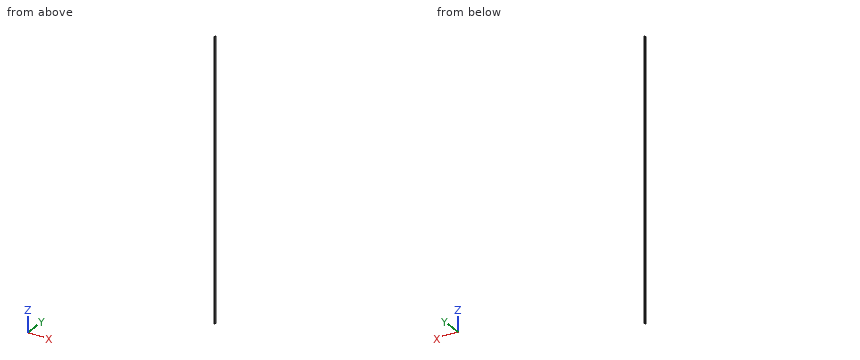
Autodesk Inventor part; units mm, degrees
ref_plane "Work Plane1" through (-1.2283, 0, 317.5) normal (0, 0, 1) x (1, 0, 0)
ref_plane "YZ Plane" through (0, 0, 0) normal (1, 0, 0) x (0, 1, 0)
ref_plane "XZ Plane" through (0, 0, 0) normal (0, 1, 0) x (-1, 0, 0)
ref_plane "Work Plane1" through (-1.2283, 0, 317.5) normal (0, 0, 1) x (1, 0, 0)
sketch "Sketch1" plane through (-1.2283, 0, 317.5) normal (0, 0, 1) x (1, 0, 0)
  line L0 (-0.3592, 8.7122) -> (-0.3592, 0.3592)
  line L1 (-0.3592, 0.3592) -> (0, 0)
  line L2 (0, 0) -> (2.4566, 0)
  line L3 (2.4566, 0) -> (2.8158, 0.3592)
  line L4 (2.8158, 0.3592) -> (2.8158, 7.6708)
  line L5 (2.8158, 7.6708) -> (2.6888, 7.6708)
  arc A0 (2.6888, 7.9248) -> (2.6888, 7.6708) centre (2.6888, 7.7978) ccw
  line L6 (2.6888, 7.9248) -> (4.3906, 7.9248)
  line L7 (4.3906, 7.9248) -> (4.3906, 8.7376)
  line L8 (4.3906, 8.7376) -> (2.2824, 10.8458)
  line L9 (2.2824, 10.8458) -> (1.7744, 10.8458)
  line L10 (1.7744, 10.8458) -> (-0.3592, 8.7122)
  point P0 (1.2283, 0)
extrude "Extrusion1" add sketch "Sketch1" against normal blind 1828.8
properties part number "vee-track"
Source: CAD feature listing. Evaluate the final solid. Frame: model axes, mm. Coordinates: 2 decimals unless noted, no trailing zeros. Loops run counter-clockwise (first coordinate to the right, second up) from the corner with the lowest first, then second, coordinate; pieces in that order, holes last. Notation, with made-up numbers: M -36,-8.75 L -10,-8.75 A20 ccw -10,-4.75 Z; hole C 21.25,52 d5. An arc over 180 degrees is marked long. Use CSV: the item, a comma, the result in double quotes.
(1) Cut plane C-C on x = -0.5. Return loops of the section in (y, z), and give its area (3 significant figures).
Answers follow:
outline,"M 0,-1511.3 L 9.8,-1511.3 L 9.8,317.5 L 0,317.5 Z"
area,"17,900 mm²"
(2) Line query: line 1 (X direction, y = 10, z = -183.5); line 2 (X direction, y = 1.5, z = -173.5); line 3 (Y direction, x = 1.5, z = -918). Output: solid intervals per line, ascending. Write a range as [from, to].
Answers follow:
line 1,"[-0.3, 1.9]"
line 2,"[-1.59, 1.59]"
line 3,"[0.27, 7.67], [7.92, 10.4]"
(3) Contact query for flat-ended pins moving along their axis: pin 1 (1 mm diameter, centred on x = -1, z = -52.5, fed in from -Y); pin 2 (6 mm diameter, centred on y = 2.5, z = -886, fed in from +X); pin 3 (0.5 mm diameter, centred on x = 2.5, z = -214.5, fed in from -Y). Output: stop coordinate, or through.
Answers follow:
pin 1,"y = 0"
pin 2,"x = 1.59"
pin 3,"y = 7.92"
(4) Cut plane A-A on z = -149.5. Return loops of the section in (x, y), and give its area (3 significant figures).
Answers follow:
outline,"M -1.59,0.36 L -1.23,0 L 1.23,0 L 1.59,0.36 L 1.59,7.67 L 1.46,7.67 A0.13 cw 1.46,7.92 L 3.16,7.92 L 3.16,8.74 L 1.05,10.85 L 0.55,10.85 L -1.59,8.71 Z"
area,"34.4 mm²"
(5) Cut plane B-B on y = 2. Return loops of the section in (x, z).
Answers follow:
outline,"M -1.59,-1511.3 L 1.59,-1511.3 L 1.59,317.5 L -1.59,317.5 Z"
